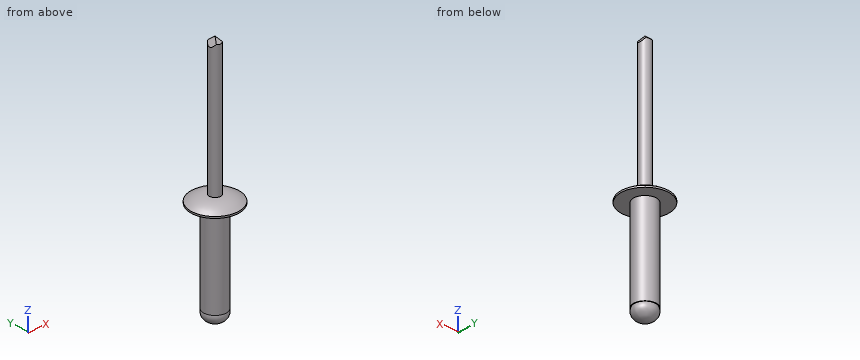
from build123d import *

# Parameters (mm, degrees)
CUT_EXTRUDE1_DEPTH      = 16.51339703
CUT_EXTRUDE1_DEPTH_BACK = 16.51339703
CUT_EXTRUDE2_DEPTH      = 16.51339703
CUT_EXTRUDE2_DEPTH_BACK = 16.51339703


with BuildPart() as part:
    # Sketch2 → Revolve1 (revolve)
    with BuildSketch(Plane(origin=(0, 0, 0), x_dir=(0, 0, -1), z_dir=(1, 0, 0)), mode=Mode.PRIVATE) as revolve1_sk:
        with BuildLine():
            Line((-15.1003, 0), (-15.1003, 0.5953125))
            Line((-15.1003, 0.5953125), (-0.8128, 0.5953125))
            ThreePointArc((-0.8128, 0.5953125), (-0.649928343, 1.606115338), (-0.1778, 2.5146))
            Line((-0.1778, 2.5146), (0, 2.5146))
            Line((0, 2.5146), (0, 1.190625))
            Line((0, 1.190625), (9.525, 1.190625))
            Line((9.525, 1.190625), (9.525, 1.122532015))
            add(Edge.make_bspline(
                [(10.7442, 0), (10.7442, 1.683798023), (9.525, 1.122532015)],
                knots=[1.570796327, 1.570796327, 1.570796327, 3.481429563, 3.481429563, 3.481429563], degree=2, weights=[1, 0.577350269, 1]))
            Line((10.7442, 0), (9.525, 0))
            Line((9.525, 0), (-15.1003, 0))
        make_face()
    revolve(revolve1_sk.sketch.rotate(Axis((0, 0, 15.1003), (0, 0, -1)), 90), axis=Axis((0, 0, 15.1003), (0, 0, -1)))

    # Sketch3 → Cut-Extrude1 (cut, two sides: drawn at the far end of the back side and taken through both)
    with BuildSketch(Plane(origin=(0, 0, 0), x_dir=(1, 0, 0), z_dir=(0, 1, 0)).offset(-CUT_EXTRUDE1_DEPTH_BACK)):
        Polygon((0, -15.1003), (0.7985125, -14.059658249), (0.7985125, -15.6083), (-0.7985125, -15.6083), (-0.7985125, -14.059658249), align=None)
    extrude(amount=CUT_EXTRUDE1_DEPTH + CUT_EXTRUDE1_DEPTH_BACK, mode=Mode.SUBTRACT)

    # Sketch5 → Cut-Extrude2 (cut, two sides: drawn at the far end of the back side and taken through both)
    with BuildSketch(Plane(origin=(0, 0, 0), x_dir=(0, 0, -1), z_dir=(1, 0, 0)).offset(-CUT_EXTRUDE2_DEPTH_BACK)):
        Polygon((-15.1003, 0), (-14.324473645, 0.9128125), (-15.4178, 0.9128125), (-15.4178, -0.9128125), (-14.324473645, -0.9128125), align=None)
    extrude(amount=CUT_EXTRUDE2_DEPTH + CUT_EXTRUDE2_DEPTH_BACK, mode=Mode.SUBTRACT)


solid = part.part
Input: part model. Units: mm. Frame: model coordinates. Coordinates: 2 decimals unless noted, no trailing zeros. Write each loop counter-clockwise with the first axis right and the second up, starting at its lowest first coordinate (ties: lowest second). Pieces come first, ordered by that corner, then holes. Notation, with made-up numbers: M 60,-38 L 67,-38 A15 ccw 67,-33 Z; hole C 47.25,-3 d5. An arc over 180 degrees is marked long. Answer as a JSON object with one key per item and string values. Group by question number.
(1) Contact query for flat-ended pins moving along their axis: P1, Ø1, axis at x = 1.5, z = -6, coming from the -Y side; P2, Ø0.7, axis at x = 0.5, y = 0, coming from the -Z side; P3, Ø2, axis at x = 1.5, y = 0.5, coming from the -Z side. Output: stop coordinate, or through.
(2) Section A-A on z = -1. Output: boundary loops of the cut face in (x, y).
(3) Section B-B on z = 5. Output: boundary loops of the cut face in (x, y), plus the area to 3 significant figures.
(4) Ray query, line 1 along X through (y, z) = (0.05, 11); line 2 along X through (y, z) = (0.5, 5.75); line 3 along Y through (x, z) = (0.7, -7.5). Return the intervals inside material, ascending. Write a range as [from, to].
Result set:
{
 "1": {"P1": "stops at y = -0.65", "P2": "stops at z = -10.74", "P3": "stops at z = -10.63"},
 "2": {"outline": "C 0,0 d2.38"},
 "3": {"outline": "C 0,0 d1.19", "area": "1.11 mm2"},
 "4": {"line 1": "x = [-0.59, 0.59]", "line 2": "x = [-0.32, 0.32]", "line 3": "y = [-0.96, 0.96]"}
}
